Source: CAD feature listing. Evaluate the final solid. Frame: model axes, mm. A direction names the side the tool comes from. Coordinates: 2 decimals unless noted, no trailing zeros. Loops run counter-clockwise (first coordinate to the right, second up) from the corner with the lowest first, then second, coordinate; pieces in that order, holes last. Notation, with made-up numbers: (-32.75, 76) -> (25.25, 76) arc R22 cw to (25.25, 93) -> close; hole circle Ø2 at (0.25, -12.75). An arc over 180 degrees is marked (long way). One line per question, with ' | ' between items. Start each with the question number.
```python
from build123d import *

# Parameters (mm, degrees)
SKETCH1_R           = 15
BOSS_EXTRUDE1_DEPTH = 40
FILLET1_R           = 10


with BuildPart() as part:
    # Sketch1 → Boss-Extrude1 (new body)
    with BuildSketch(Plane(origin=(0, 0, 0), x_dir=(0, 0, -1), z_dir=(1, 0, 0))):
        with BuildLine():
            ThreePointArc((132.694646831, -65.009266851), (168.499781041, -100.12380247), (132.447129149, -134.984160172))
            ThreePointArc((132.447129149, -134.984160172), (59.3634858, -117.047102518), (0, -70.79849696))
            ThreePointArc((0, -70.79849696), (-59.3634858, -117.047102518), (-132.447129149, -134.984160172))
            ThreePointArc((-132.447129149, -134.984160172), (-168.499781041, -100.12380247), (-132.694646831, -65.009266851))
            ThreePointArc((-132.694646831, -65.009266851), (-70.44161018, -45.071700409), (-33.805757942, 9.064807223))
            ThreePointArc((-33.805757942, 9.064807223), (0, 35), (33.805757942, 9.064807223))
            ThreePointArc((33.805757942, 9.064807223), (70.44161018, -45.071700409), (132.694646831, -65.009266851))
        make_face()
        Circle(SKETCH1_R, mode=Mode.SUBTRACT)
        with Locations((-133.5, -100)):
            Circle(SKETCH1_R, mode=Mode.SUBTRACT)
        with Locations((133.5, -100)):
            Circle(SKETCH1_R, mode=Mode.SUBTRACT)
    extrude(amount=BOSS_EXTRUDE1_DEPTH)

    # Fillet1
    fillet1_edges = [part.edges().sort_by_distance(p)[0] for p in [
        (0, -117.047102518, -59.3634858),
        (0, -117.047102518, 59.3634858),
        (0, -100.12380247, 168.499781041),
        (0, -45.071700409, 70.44161018),
        (0, 35, 0),
        (0, -45.071700409, -70.44161018),
        (0, -100.12380247, -168.499781041),
        (40, -100.12380247, -168.499781041),
        (40, -45.071700409, -70.44161018),
        (40, 35, 0),
        (40, -45.071700409, 70.44161018),
        (40, -100.12380247, 168.499781041),
        (40, -117.047102518, 59.3634858),
        (40, -117.047102518, -59.3634858),
    ]]
    fillet(fillet1_edges, radius=FILLET1_R)


solid = part.part
```
(1) Ray query, L1, parallel to Y at x = 23, z = 133.5; L2, parallel to Z at x = 20, y = -105.5; L3, parallel to Z at x = 12.5, y = 7. Return the intervals inside material, ascending.
(2) Cut plane A-A, the plane x = 36. Return the cut outline in (y, z).
(3) Draft query along Y for faces 1 (the cylindrical face through (19.86, -44.51, -69.7)), 2 (the cylindrical face through (19.72, -114.643, 136.752)), 3 (the cylindrical face through (19.86, -100.91, 168.49)), 4 (the cylindrical face through (19.72, 0.66, 14.985)). Return one class per face: pulls with the +Y half, pulls with the -Y half, needs draft (parallel to the pull), parting line crosses it, or undercut.
(4) Contact query for flat-ended pins moving along their axis: pin 1 Ø4 at (x, z) = (16.5, -116.5) entering from -Y; pin 2 Ø18 at (y, z) = (-100, -133.5) entering from +X; pin 3 Ø1.5 at (y, z) = (-110, 59.5) entering from +X; pin 4 Ø12 at (x, z) = (15, -36.5) entering from +Y. Output: stop coordinate, or through.
(5) Cut plane B-B, the plane y = -100. State how many separate pieces and enclosed holes the cut face has, and give its area (3 significant figures).
(6) Access query for faces 5 (the cylindrical face through (19.72, -114.643, -130.248)), 6 (the cylindrical face through (19.86, -116.58, 58.41)). Directions: +Z, -Z, +X, -X, +Y, -Y. A direction counts if a zero-diameter tool reaches every point of the face in a straight line with its end or side. Return the directions, or none.
Here are the results:
1) L1: y = -135 to -115, -85 to -65 | L2: z = -168.07 to -147.46, -119.54 to -39.02, 39.02 to 119.54, 147.46 to 168.07 | L3: z = -34.38 to -13.27, 13.27 to 34.38
2) outline: (-132.99, -132.51) arc R33 ccw (long way) to (-67.01, -132.74) arc R102 cw to (8.55, -31.87) arc R33 ccw to (8.55, 31.87) arc R102 cw to (-67.01, 132.74) arc R33 ccw (long way) to (-132.99, 132.51) arc R178 ccw to (-67.66, 0) arc R178 ccw to start; hole circle Ø30 at (-100, -133.5); hole circle Ø30 at (-100, 133.5); hole circle Ø30 at (0, 0)
3) face 1: pulls with the +Y half | face 2: undercut | face 3: parting line crosses it | face 4: undercut
4) pin 1: stops at y = -134.02 | pin 2: passes through | pin 3: stops at x = 39.58 | pin 4: stops at y = 17.17
5) separate pieces: 4 | enclosed holes: 0 | area: 8,360 mm2
6) face 5: +X, -X | face 6: +X, -X, -Y
